```python
from build123d import *

# Parameters (mm, degrees)
F1_DEPTH      = 3
F2_W          = 4
F2_H          = 6.1803398875
F3_DEPTH      = 1
F5_DEPTH      = 10.001
F5_DEPTH_BACK = 8.0911699437
F6_R          = 0.5
F7_T1_DEPTH   = 13.5993141484
F8_DEPTH      = 1


# Not quite as in the source:
# - a fillet or chamfer that OpenCascade refuses, or shapes differently, is made with other operations: its cross-section is extruded or revolved along the edge and cut away or added


with BuildPart() as f1:
    # F0 (on Top) → F1 (new body)
    with BuildSketch(Plane.XY):
        Polygon((3.63271264, -1.1803398875), (9.510565163, 3.0901699437), (2.2451398829, 3.0901699437), align=None)
        Polygon((3.63271264, -1.1803398875), (2.2451398829, 3.0901699437), (-2.2451398829, 3.0901699437), (-3.63271264, -1.1803398875), (0, -3.8196601125), align=None)
        Polygon((-2.2451398829, 3.0901699437), (2.2451398829, 3.0901699437), (0, 10), align=None)
        Polygon((5.8778525229, -8.0901699437), (3.63271264, -1.1803398875), (0, -3.8196601125), align=None)
        Polygon((-3.63271264, -1.1803398875), (-2.2451398829, 3.0901699437), (-9.510565163, 3.0901699437), align=None)
        Polygon((-5.8778525229, -8.0901699437), (0, -3.8196601125), (-3.63271264, -1.1803398875), align=None)
    extrude(amount=F1_DEPTH)

    # F2 (on face) → F3 (join)
    with BuildSketch(Plane.XY.offset(3)):
        Polygon((3.63271264, -1.1803398875), (9.510565163, 3.0901699437), (2.2451398829, 3.0901699437), (0, 10), (-2.2451398829, 3.0901699437), (-9.510565163, 3.0901699437), (-3.63271264, -1.1803398875), (-5.8778525229, -8.0901699437), (0, -3.8196601125), (5.8778525229, -8.0901699437), align=None)
        Rectangle(F2_W, F2_H, mode=Mode.SUBTRACT)
        Rectangle(F2_W, F2_H)
    extrude(amount=F3_DEPTH)

    # F4 (on Front) → F5 (cut, two sides)
    with BuildSketch(Plane.XZ) as f5_sk:
        with BuildLine():
            ThreePointArc((-0.75, 3.7348469228), (-0.3968626967, 2.0278888952), (1.05, 3))
            ThreePointArc((1.05, 3), (0.9721111048, 3.3968626967), (0.75, 3.7348469228))
            ThreePointArc((0.75, 3.7348469228), (0, 4.05), (-0.75, 3.7348469228))
        make_face()
        with BuildLine():
            ThreePointArc((-0.75, 3.7348469228), (0, 4.05), (0.75, 3.7348469228))
            Line((0.75, 3.7348469228), (0.75, 5))
            Line((0.75, 5), (-0.75, 5))
            Line((-0.75, 5), (-0.75, 3.7348469228))
        make_face()
    extrude(amount=-F5_DEPTH, mode=Mode.SUBTRACT)
    extrude(f5_sk.sketch, amount=F5_DEPTH_BACK, mode=Mode.SUBTRACT)

    # F6
    f6_edges = [f1.edges().sort_by_distance(p)[0] for p in [
        (5.877853, -8.09017, 2),
        (9.510565, 3.09017, 2),
        (0, 10, 0.975),
        (-9.510565, 3.09017, 2),
        (-5.877853, -8.09017, 2),
    ]]
    fillet(f6_edges, radius=F6_R)

    # F7: chamfer of 0.3 on 2 edges, made by hand

    # F7_s2 → F7_t1 (cut)
    with BuildSketch(Plane.XZ.offset(-8.4632422435)):
        Polygon((-0.75, 3.7), (-1.05, 4), (-0.75, 4), align=None)
        Polygon((1.05, 4), (0.75, 3.7), (0.75, 4), align=None)
    extrude(amount=F7_T1_DEPTH, mode=Mode.SUBTRACT)

    # F8 (cut): a face of the model
    f8_faces = [f1.faces().sort_by_distance(p)[0] for p in [
        (0, 0, 0),
    ]]
    extrude(f8_faces, amount=-F8_DEPTH, mode=Mode.SUBTRACT)


solid = f1.part
```
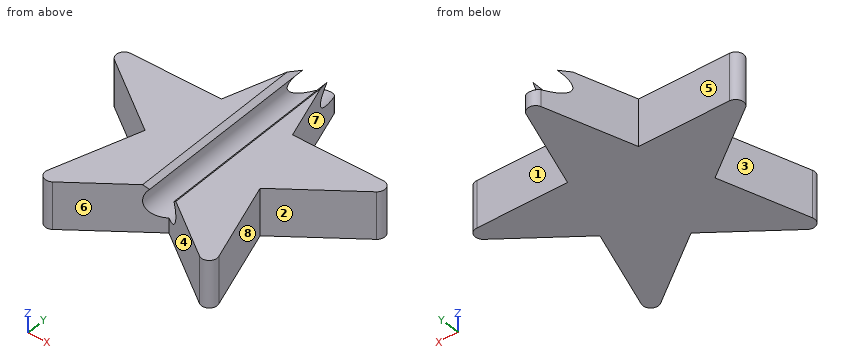
Can you work these out from the model? Positions are in its coordinate system, mm. Face numbers are marked on the shaded views. A direction names the side the tool comes from. Coordinates: 2 decimals unless noted, no trailing zeros. Order: outer loops, then holes, each group sorted by start corner. A loop starts at its lowest first (then second) coordinate and runs counter-clockwise, first axis right, second up.
1. If we section it at C-C (z = 1.4): Please give me the cut outline in (x, y), then the cut area to 3 significant figures.
2. For the marked faces 1, 2, 3, 4 and 5, which set-ups out of +Z, -Z, +X, -X, +Y, -Y let a thin tool reach every point of the face, with its end or its side?
3. Thinking about a two-plate mould opening in Y: for the marked faces 6, 7 and 8, which applies, +Y half, -Y half, draft (parallel to the pull), parting line (faces both ways), or undercut?
4. If we section it at D-D (y = 1.5): Please give me the cut outline in (x, z).
5. I need wall thicknesses on line 1 (X direction, y = 4.5, z = 3.5); line 2 (X direction, y = 2, z = 3); line 3 (Y direction, x = 5.5, z = 1.4). Which ranges of each line are inside material? Lowest first, please.
6. If we section it at B-B (y = -5): Please give me the cut outline in (x, z).
7. If we section it at A-A (z = 3): Please give me the cut outline in (x, y), then the cut area to 3 significant figures.
8. I'm going to push flat-ended pins straight in: pin 1 (1.5 mm diameter, centred on y = -3.5, z = 2, fed in from -X); pin 2 (0.9 mm diameter, centred on x = 6, z = 2.5, fed in from +Y). Where does each tip first touch, or does it pass through?
Entries:
1. outline: (-8.27, 2.19) - (-3.63, -1.18) - (-5.4, -6.63) arc R0.5 ccw to (-4.63, -7.19) - (0, -3.82) - (4.63, -7.19) arc R0.5 ccw to (5.4, -6.63) - (3.63, -1.18) - (8.27, 2.19) arc R0.5 ccw to (7.97, 3.09) - (2.25, 3.09) - (0.48, 8.54) arc R0.5 ccw to (-0.48, 8.54) - (-2.25, 3.09) - (-7.97, 3.09) arc R0.5 ccw to start
1. area: 110 mm2
2. face 1: +Z, -Z, +X, +Y
2. face 2: +Z, -Z, +X
2. face 3: +Z, -Z, -X
2. face 4: +Z, -Z, -Y
2. face 5: +Z, -Z, -X, +Y
3. face 6: -Y half
3. face 7: +Y half
3. face 8: undercut
4. outline: (-7.32, 1) - (7.32, 1) - (7.32, 4) - (1.05, 4) - (0.77, 3.72) arc R1.05 cw (long way) to (-0.77, 3.72) - (-1.05, 4) - (-7.32, 4) - close
5. line 1: x = -1.79 to -0.92, 0.92 to 1.79
5. line 2: x = -8.01 to -1.05, 1.05 to 8.01
5. line 3: y = 0.18 to 3.09
6. outline: (-4.87, 1) - (-1.62, 1) - (-1.62, 4) - (-4.87, 4) - close; (1.62, 1) - (4.87, 1) - (4.87, 4) - (1.62, 4) - close
7. outline: (-8.27, 2.19) - (-3.63, -1.18) - (-5.4, -6.63) arc R0.5 ccw to (-4.63, -7.19) - (-1.05, -4.58) - (-1.05, 6.77) - (-2.25, 3.09) - (-7.97, 3.09) arc R0.5 ccw to start; (1.05, -4.58) - (4.63, -7.19) arc R0.5 ccw to (5.4, -6.63) - (3.63, -1.18) - (8.27, 2.19) arc R0.5 ccw to (7.97, 3.09) - (2.25, 3.09) - (1.05, 6.77) - close
7. area: 84.0 mm2
8. pin 1: stops at x = -4.63
8. pin 2: stops at y = 3.09
